from build123d import *

# Parameters (mm, degrees)
F1_DEPTH = 2.75
F2_W     = 4.75
F2_H     = 1
F3_DEPTH = 1
F4_D     = 0.5
F4_DEPTH = 2.75
F4_TIP   = 0.1502151548
F5_R     = 5
F5_R_2   = 1.2515883102
F5_R_3   = 0.25
F6_DEPTH = 0.5


with BuildPart() as f1:
    # F0 (on Top) → F1 (new body)
    with BuildSketch(Plane.XY):
        Polygon((61.25, -53.875), (61.25, 53.875), (2.7548319194, 53.875), (-2.7548319194, 53.875), (-61.25, 53.875), (-61.25, -53.875), align=None)
        with BuildLine():
            Line((-2.7548319194, 53.875), (2.7548319194, 53.875))
            ThreePointArc((2.7548319194, 53.875), (0, 56.6298319194), (-2.7548319194, 53.875))
        make_face()
    extrude(amount=F1_DEPTH)

    # F2 (on face) → F3 (join)
    with BuildSketch(Plane.XZ.offset(53.875)):
        with Locations((-49, 0.5)):
            Rectangle(F2_W, F2_H)
        with Locations((49, 0.5)):
            Rectangle(F2_W, F2_H)
    extrude(amount=F3_DEPTH)

    # F4
    with Locations(Plane(origin=(0, 0, 0), x_dir=(1, 0, 0), z_dir=(0, 0, -1))):
        with Locations((0, -53.875)):
            Hole(F4_D / 2, depth=F4_DEPTH)
            with Locations((0, 0, -(F4_DEPTH + F4_TIP / 2))):  # 118° drill point
                Cone(0, F4_D / 2, F4_TIP, mode=Mode.SUBTRACT)

    # F5 (on face) → F6 (cut)
    with BuildSketch(Plane.XY.offset(2.75)):
        with Locations((51.25, 43.875)):
            Circle(F5_R)
        with Locations((-0.0143809427, 53.9503525943)):
            Circle(F5_R_2)
        with Locations((0, 53.875)):
            Circle(F5_R_3, mode=Mode.SUBTRACT)
        with Locations((-51.25, 43.875)):
            Circle(F5_R)
        with Locations((51.25, -43.875)):
            Circle(F5_R)
        with Locations((-51.25, -43.875)):
            Circle(F5_R)
    extrude(amount=-F6_DEPTH, mode=Mode.SUBTRACT)


solid = f1.part
Input: part model. Units: mm. Frame: model coordinates. A direction names the side the tool comes from. Round coordinates to 2 decimals unless told otherwise and drop trailing zeros. Order: outer loops, then holes, each group sorted by start corner. A loop starts at its lowest first (then second) coordinate and runs counter-clockwise, first axis right, second up.
1. Cut plane A-A, the plane z = 0.5. Output: boundary loops of the cut face in (x, y) (3 decimals).
The answers:
outline: (-61.25, -53.875) - (-51.375, -53.875) - (-51.375, -54.875) - (-46.625, -54.875) - (-46.625, -53.875) - (46.625, -53.875) - (46.625, -54.875) - (51.375, -54.875) - (51.375, -53.875) - (61.25, -53.875) - (61.25, 53.875) - (2.755, 53.875) arc R2.755 ccw to (-2.755, 53.875) - (-61.25, 53.875) - close; hole circle Ø0.5 at (0, 53.875)
2. Pin query (flat end, axial travel): P1, Ø9, axis at x = 51.25, y = -43.875, coming from the +Z side; P2, Ø1.4, axis at x = -43, z = 1.5, coming from the +Y side (3 decimals); P3, Ø1.1, axis at x = 48, y = -54.5, coming from the +Z side. Return the tip coordinate at first contact, or that it passes through.
The answers:
P1: stops at z = 2.25
P2: stops at y = 53.875
P3: stops at z = 1
3. Set-up query: faces 1 (the face through (32, 53.875, 1)), 2 (the face through (-1, 2, 0)), 3 (the face through (50.599, 48.832, 2.504)). Return all of +Z, -Z, +X, -X, +Y, -Y with unobstructed straight access to the full face (end or side cutting, diameter ignored); none if empty.
The answers:
face 1: +Z, -Z, +X, +Y
face 2: -Z, +X, -X, +Y, -Y
face 3: +Z
4. Material intervals for line 1 (Y direction, x = -51.25, z = 2.4) (3 decimals); line 2 (Y direction, x = -16.5, z = 0.4) (3 decimals); line 3 (Z direction, x = -54, y = -46), sorted ascending.
The answers:
line 1: y = -53.875 to -48.875, -38.875 to 38.875, 48.875 to 53.875
line 2: y = -53.875 to 53.875
line 3: z = 0 to 2.25
5. Mould query, pull axis Y, two halves, no side actions, for faces 4 (the face through (-0.29, 52.73, 2.5)), 5 (the face through (-32, 53.875, 1)), 6 (the face through (-1, 2, 2.75)). Classes: released by +Y, released by -Y, zero draft, split by the parting line, or undercut.
The answers:
face 4: undercut
face 5: released by +Y
face 6: zero draft
